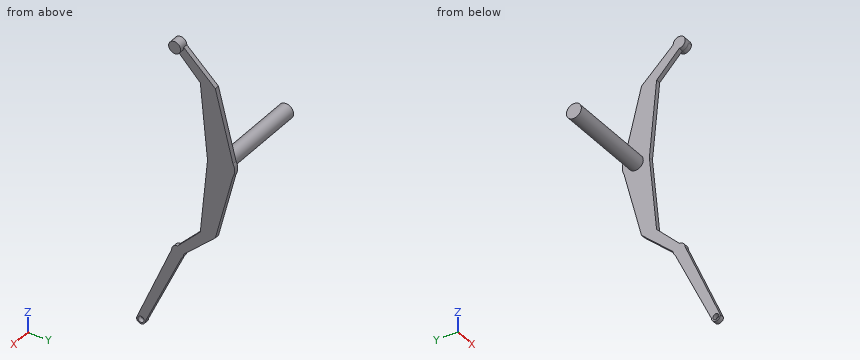
from build123d import *

# Parameters (mm, degrees)
SKETCH1_R           = 20
BOSS_EXTRUDE1_DEPTH = 30
BOSS_EXTRUDE2_DEPTH = 60
SKETCH1_4_R         = 49.5
BOSS_EXTRUDE3_DEPTH = 600


with BuildPart() as part:
    # Sketch1 → Boss-Extrude1 (new body)
    with BuildSketch(Plane(origin=(0, 0, 0), x_dir=(0, 0, -1), z_dir=(1, 0, 0))):
        with BuildLine():
            Line((-500, -38.163490354), (-693.137754961, -248.163490354))
            ThreePointArc((-693.137754961, -248.163490354), (-721.652707583, -316.215183298), (-653.1431202, -288.818616504))
            Line((-653.1431202, -288.818616504), (-500, -138.163490354))
            Line((-500, -138.163490354), (0, -90))
            Line((0, -90), (500, -138.163490354))
            Line((500, -138.163490354), (653.1431202, -288.818616504))
            ThreePointArc((653.1431202, -288.818616504), (665.086062018, -316.678442975), (693.137754961, -328.163490354))
            Line((693.137754961, -328.163490354), (1241.260569265, -562.203490354))
            ThreePointArc((1241.260569265, -562.203490354), (1271.260569265, -532.203490354), (1241.260569265, -502.203490354))
            Line((1241.260569265, -502.203490354), (723.659328701, -262.309408733))
            ThreePointArc((723.659328701, -262.309408733), (709.957932356, -251.87187104), (693.137754961, -248.163490354))
            Line((693.137754961, -248.163490354), (500, -38.163490354))
            Line((500, -38.163490354), (43.294270514, 78.902510357))
            ThreePointArc((43.294270514, 78.902510357), (0, 90), (-43.294270514, 78.902510357))
            Line((-43.294270514, 78.902510357), (-500, -38.163490354))
        make_face()
        with Locations((1241.260569265, -532.203490354)):
            Circle(SKETCH1_R, mode=Mode.SUBTRACT)
    extrude(amount=BOSS_EXTRUDE1_DEPTH)

    # Sketch1_3 → Boss-Extrude2 (add)
    with BuildSketch(Plane(origin=(0, 0, 0), x_dir=(0, 0, -1), z_dir=(1, 0, 0))):
        with BuildLine():
            ThreePointArc((-653.137754961, -288.163490354), (-664.853483714, -259.879219107), (-693.137754961, -248.163490354))
            ThreePointArc((-693.137754961, -248.163490354), (-733.137754961, -288.163490354), (-693.137754961, -328.163490354))
            Line((-693.137754961, -328.163490354), (-653.1431202, -288.818616504))
            ThreePointArc((-653.1431202, -288.818616504), (-653.139096293, -288.491064414), (-653.137754961, -288.163490354))
        make_face()
        with BuildLine():
            Line((-653.1431202, -288.818616504), (-693.137754961, -328.163490354))
            ThreePointArc((-693.137754961, -328.163490354), (-665.086062018, -316.678442975), (-653.1431202, -288.818616504))
        make_face()
    extrude(amount=BOSS_EXTRUDE2_DEPTH)

    # Sketch1_4 → Boss-Extrude3 (add)
    with BuildSketch(Plane(origin=(0, 0, 0), x_dir=(0, 0, -1), z_dir=(1, 0, 0))):
        Circle(SKETCH1_4_R)
    extrude(amount=-BOSS_EXTRUDE3_DEPTH)


solid = part.part
Verification items for the finished model (mm, model axes). Give positions to 0.01 mm unless a question says otherwise; leave off trailing zeros. Loops run counter-clockwise (first coordinate to the right, second up) from the corner with the lowest first, then second, coordinate; pieces in that order, holes last. Notation, with made-up numbers: (-29.75, -30) - (-7.75, -30) arc R17 cw to (-7.75, 3) - close; hole circle Ø1 at (-30, 69.5). An arc over 180 degrees is marked (long way). Write item = value, one per line. Start each with the question number.
Q1. Cross-section at B-B, the plane x = -472. Enter the section's corners in (y, z).
Q2. Depth check by flat-ended pin: P1, Ø12, axis at x = -407.5, y = 0, coming from the -Z side; P2, Ø8, axis at x = -357, z = 4, coming from the +Y side; P3, Ø24, axis at y = -532.2, z = -1241.26, coming from the -X side. Enter the tip coordinate at first touch or a pass-through.
Q3. Cross-section at D-D, the plane y = -416.5. Enter the section's corners in (x, z).
Q4. Thickness scan on line 1 (X direction, y = -14, z = -274); line 2 (Z direction, x = 15, y = -526); line 3 (Z direction, x = -175, y = -29). Record the ranges inside material, lowest first.
Q5. Cross-section at A-A, the plane y = 0. Enter the section's corners in (x, z), and give its area (3 significant figures).
Q6. Cross-section at C-C, the plane z = -1141. Enter the section's corners in (x, y), and give its area (3 significant figures).
Answer key:
q1.outline = circle Ø99 at (0, 0)
q2.P1 = -49.5
q2.P2 = 49.5
q2.P3 = through
q3.outline = (0, -1056.34) - (30, -1056.34) - (30, -900.02) - (0, -900.02) - close
q4.line_1 = 0 to 30
q4.line_2 = -1270.61 to -1260.27, -1222.25 to -1156.47
q4.line_3 = -40.12 to 40.12
q5.outline = (-600, -49.5) - (0, -49.5) - (0, -351.11) - (30, -351.11) - (30, 351.11) - (0, 351.11) - (0, 49.5) - (-600, 49.5) - close
q5.area = 80,500 mm^2
q6.outline = (0, -519.39) - (30, -519.39) - (30, -455.74) - (0, -455.74) - close
q6.area = 1,910 mm^2
